Geometry: final body of the model. Coordinates: model frame, mm. Give positions to 0.01 mm unless a question says otherwise; leave off trailing zeros. Write each loop counter-clockwise with the first axis right and the second up, starting at its lowest first coordinate (ties: lowest second). Pieces come first, ordered by that corner, then holes.
Q1. Cut plane D-D on z = 0.95. Count the separate pieces of the cut face and the enclosed holes in it, plus the area to 3 significant figures.
Q2. Cut plane C-C on x = -10. Return the cut outline in (y, z), plus the area to 3 significant figures.
Q3. Cut plane A-A on x = -41. Return the cut outline in (y, z).
Q4. Line query: L1, parallel to Y at x = 0, z = 1.3; L2, parallel to Y at x = -10, z = 1.4; L3, parallel to X at y = -12.5, z = 1.75. Output: solid intervals per line, ascending.
Q5. Pin query (flat end, axial travel): pin 1 (3 mm diameter, centred on x = -59.73, y = 3.45, fed in from -Z); pin 2 (8 mm diameter, centred on x = -28, y = 19, fed in from -Z); pin 3 (1 mm diameter, centred on y = -71.5, z = 0.5, fed in from +X). Return the tip coordinate at first contact, or that it passes through.
Q6. Draft query along X for faces 1 (the face through (-13, -24, 2)), 2 (the face through (-18.35, -22.24, 0.99)). Return one class per face: pulls with the +X half, pulls with the -X half, needs draft (parallel to the pull), parting line crosses it, or undercut.
Q7. Cut plane B-B on y = 0. Return the cut outline in (x, z), plus the area to 3 significant figures.
```python
from build123d import *

# Parameters (mm, degrees)
ESQUISSE1_W             = 19
ESQUISSE1_H             = 70
ESQUISSE1_R             = 1.7
BOSS_EXTRU_1_DEPTH      = 2
BOSS_EXTRU_2_DEPTH      = 2
ESQUISSE3_R             = 1.7
ESQUISSE3_R_2           = 1
ESQUISSE3_W             = 34.416616224
ESQUISSE3_H             = 3.721706088
ESQUISSE3_H_2           = 3.894041755
ESQUISSE3_H_3           = 3.892627661
ESQUISSE3_W_2           = 33.600664609
ESQUISSE3_H_4           = 3.878874163
ESQUISSE3_H_5           = 3.860536167
ESQUISSE3_H_6           = 3.860536168
ESQUISSE3_W_3           = 4.02824374
ENL_V_MAT_EXTRU_1_DEPTH = 2
ESQUISSE4_R             = 1.7
ENL_V_MAT_EXTRU_2_DEPTH = 2


with BuildPart() as part:
    # Esquisse1 → Boss.-Extru.1 (new body)
    with BuildSketch(Plane.XY):
        with Locations((-2.5, -24.85)):
            Rectangle(ESQUISSE1_W, ESQUISSE1_H)
        Circle(ESQUISSE1_R, mode=Mode.SUBTRACT)
        with Locations((0, -49.7)):
            Circle(ESQUISSE1_R, mode=Mode.SUBTRACT)
    extrude(amount=BOSS_EXTRU_1_DEPTH)

    # Esquisse2 → Boss.-Extru.2 (add)
    with BuildSketch(Plane(origin=(0, 0, 0), x_dir=(-1, 0, 0), z_dir=(0, 0, -1))):
        Polygon((67.5, -22.717620887), (67.5, 40.15), (2.5, 40.15), (2.5, -89.85), (67.5, -89.85), (67.5, -26.982379113), align=None)
    extrude(amount=-BOSS_EXTRU_2_DEPTH)

    # Esquisse3 → Enlèv. mat.-Extru.1 (cut)
    with BuildSketch(Plane(origin=(0, 0, 0), x_dir=(-1, 0, 0), z_dir=(0, 0, -1))):
        with Locations((16.729252348, -41.85)):
            Circle(ESQUISSE3_R)
        with Locations((16.729252348, -66.968565228)):
            Circle(ESQUISSE3_R_2)
        with Locations((54.029252348, -66.968565228)):
            Circle(ESQUISSE3_R_2)
        with Locations((16.729252348, -22.75)):
            Circle(ESQUISSE3_R)
        with Locations((16.729252348, -10.75)):
            Circle(ESQUISSE3_R)
        with Locations((16.729252348, 4.25)):
            Circle(ESQUISSE3_R)
        with Locations((16.729252348, 16.25)):
            Circle(ESQUISSE3_R)
        with Locations((16.729252348, 37.25)):
            Circle(ESQUISSE3_R)
        with Locations((59.729252348, -41.85)):
            Circle(ESQUISSE3_R)
        with Locations((59.729252348, -21.55)):
            Circle(ESQUISSE3_R)
        with Locations((59.729252348, -10.75)):
            Circle(ESQUISSE3_R)
        with Locations((59.729252348, 3.45)):
            Circle(ESQUISSE3_R)
        with Locations((37.636895851, -39.989146956)):
            Rectangle(ESQUISSE3_W, ESQUISSE3_H)
        with Locations((37.636895851, -24.697020878)):
            Rectangle(ESQUISSE3_W, ESQUISSE3_H_2)
        with Locations((37.636895851, -11.228994179)):
            Rectangle(ESQUISSE3_W, ESQUISSE3_H_3)
        with Locations((37.228920043, 4.281571073)):
            Rectangle(ESQUISSE3_W_2, ESQUISSE3_H_4)
        with Locations((37.228920043, 16.012867078)):
            Rectangle(ESQUISSE3_W_2, ESQUISSE3_H_5)
        with Locations((37.228920043, 37.153497731)):
            Rectangle(ESQUISSE3_W_2, ESQUISSE3_H_6)
        with Locations((65.48587813, -11.228994179)):
            Rectangle(ESQUISSE3_W_3, ESQUISSE3_H_3)
    extrude(amount=-ENL_V_MAT_EXTRU_1_DEPTH, mode=Mode.SUBTRACT)

    # Esquisse4 → Enlèv. mat.-Extru.2 (cut)
    with BuildSketch(Plane(origin=(0, 0, 0), x_dir=(-1, 0, 0), z_dir=(0, 0, -1))):
        with Locations((10, -49.7)):
            Circle(ESQUISSE4_R)
        with Locations((10, 0)):
            Circle(ESQUISSE4_R)
    extrude(amount=-ENL_V_MAT_EXTRU_2_DEPTH, mode=Mode.SUBTRACT)


solid = part.part
```
Data:
1. separate pieces: 1
1. enclosed holes: 22
1. area: 8,180 mm2
2. outline: (-89.85, 0) - (-51.4, 0) - (-51.4, 2) - (-89.85, 2) - close; (-48, 0) - (-1.7, 0) - (-1.7, 2) - (-48, 2) - close; (1.7, 0) - (40.15, 0) - (40.15, 2) - (1.7, 2) - close
2. area: 246 mm2
3. outline: (-89.85, 0) - (-41.85, 0) - (-41.85, 2) - (-89.85, 2) - close; (-38.13, 0) - (-26.64, 0) - (-26.64, 2) - (-38.13, 2) - close; (-22.75, 0) - (-13.18, 0) - (-13.18, 2) - (-22.75, 2) - close; (-9.28, 0) - (2.34, 0) - (2.34, 2) - (-9.28, 2) - close; (6.22, 0) - (14.08, 0) - (14.08, 2) - (6.22, 2) - close; (17.94, 0) - (35.22, 0) - (35.22, 2) - (17.94, 2) - close; (39.08, 0) - (40.15, 0) - (40.15, 2) - (39.08, 2) - close
4. L1: y = -59.85 to -51.4, -48 to -1.7, 1.7 to 10.15
4. L2: y = -89.85 to -51.4, -48 to -1.7, 1.7 to 40.15
4. L3: x = -63.47 to -54.85, -20.43 to 7
5. pin 1: passes through
5. pin 2: stops at z = 0
5. pin 3: stops at x = -2.5
6. face 1: needs draft
6. face 2: undercut
7. outline: (-67.5, 0) - (-11.7, 0) - (-11.7, 2) - (-67.5, 2) - close; (-8.3, 0) - (-1.7, 0) - (-1.7, 2) - (-8.3, 2) - close; (1.7, 0) - (7, 0) - (7, 2) - (1.7, 2) - close
7. area: 135 mm2
